Verification items for the finished model (mm, model axes). Face numbers are marked on the shaded views. A direction names the side the tool comes from. Round coordinates to 2 decimals unless told otherwise and drop trailing zeros. Order: outer loops, then holes, each group sorted by start corner. A loop starts at its lowest first (then second) coordinate and runs counter-clockwise, first axis right, second up. Notation, with made-up numbers: (47, 55.25) -> (63, 55.25) arc R8 ccw to (63, 65.25) -> close; hole circle Ø11 at (69.25, 81). An arc over 180 degrees is marked (long way). Return JSON: item names as keys, results as strings. Group by question number.
Item 1: Sectioned sample at B-B on z = 11.5. Give the number of separate pieces and of enclosed holes in the cut face, plus the area to 3 significant figures.
Item 2: Sectioned sample at D-D on y = -11.5. Record the cut outline in (x, z).
Item 3: Draft check along Y on the marked faces 1, 2 and 3. Enter one of: pulls with the +Y half, pulls with the -Y half, needs draft (parallel to the pull), parting line crosses it, or undercut.
Item 4: Access from +Z, -Z, +X, -X, +Y, -Y to the whole of each face (thin tool, end or side, straight path). Record for the marked faces 4 and 5.
Item 5: Sectioned sample at C-C on y = -6. Record the cut outline in (x, z).
Item 6: Sectioned sample at A-A on x = -2. Record the cut outline in (y, z), plus the area to 3 significant figures.
Item 7: Depth check by flat-ended pin: pin 1 Ø2 at (y, z) = (9.5, 6) entering from +X; pin 2 Ø1 at (x, z) = (-8.5, 11) entering from -Y; pin 3 Ø2 at (x, z) = (-11.5, 11.5) entering from -Y. Enter the tip coordinate at first touch or a pass-through.
Item 8: Scan lines: probe 1 along Y at (x, z) = (6.5, 6); probe 2 along Y at (x, z) = (-2, 10); probe 3 along X at (y, z) = (-7.5, 7.75). Record each from-to range of solid material in increasing order. Write a range as from..to.
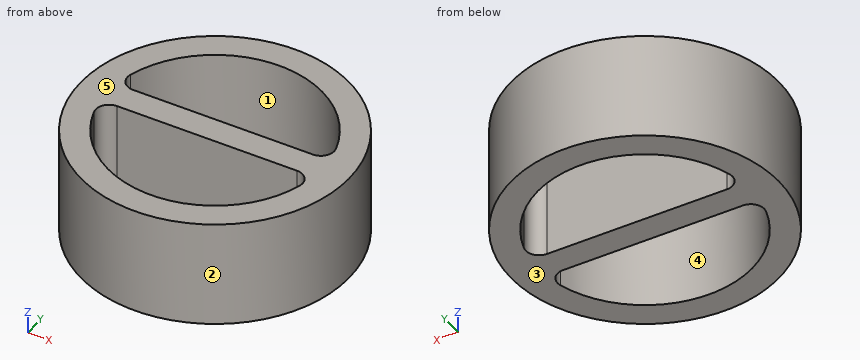
```python
from build123d import *

# Parameters (mm, degrees)
F1_DEPTH = 12.7


with BuildPart() as f1:
    # F0 (on Top) → F1 (new body)
    with BuildSketch(Plane.XY):
        with BuildLine():
            Line((-15.875, 0), (15.875, 0))
            ThreePointArc((15.875, 0), (0, 15.875), (-15.875, 0))
        make_face()
        with BuildLine():
            Line((10.649274, 1.5875), (-10.649274, 1.5875))
            ThreePointArc((-10.649274, 1.5875), (-11.922105, 2.226287), (-12.170599, 3.628571))
            ThreePointArc((-12.170599, 3.628571), (0, 12.7), (12.170599, 3.628571))
            ThreePointArc((12.170599, 3.628571), (11.922105, 2.226287), (10.649274, 1.5875))
        make_face(mode=Mode.SUBTRACT)
        with BuildLine():
            ThreePointArc((-15.875, 0), (0, -15.875), (15.875, 0))
            Line((15.875, 0), (-15.875, 0))
        make_face()
        with BuildLine():
            ThreePointArc((12.170599, -3.628571), (0, -12.7), (-12.170599, -3.628571))
            ThreePointArc((-12.170599, -3.628571), (-11.922105, -2.226287), (-10.649274, -1.5875))
            Line((-10.649274, -1.5875), (10.649274, -1.5875))
            ThreePointArc((10.649274, -1.5875), (11.922105, -2.226287), (12.170599, -3.628571))
        make_face(mode=Mode.SUBTRACT)
    extrude(amount=F1_DEPTH)


solid = f1.part
```
Recorded:
{
 "1": {"separate pieces": "1", "enclosed holes": "2", "area": "369 mm²"},
 "2": {"outline": "(-10.94, 0) -> (-5.39, 0) -> (-5.39, 12.7) -> (-10.94, 12.7) -> close; (5.39, 0) -> (10.94, 0) -> (10.94, 12.7) -> (5.39, 12.7) -> close"},
 "3": {"face 1": "undercut", "face 2": "parting line crosses it", "face 3": "needs draft"},
 "4": {"face 4": "+Z, -Z", "face 5": "+Z, +X, -X, +Y, -Y"},
 "5": {"outline": "(-14.7, 0) -> (-11.19, 0) -> (-11.19, 12.7) -> (-14.7, 12.7) -> close; (11.19, 0) -> (14.7, 0) -> (14.7, 12.7) -> (11.19, 12.7) -> close"},
 "6": {"outline": "(-15.75, 0) -> (-12.54, 0) -> (-12.54, 12.7) -> (-15.75, 12.7) -> close; (-1.59, 0) -> (1.59, 0) -> (1.59, 12.7) -> (-1.59, 12.7) -> close; (12.54, 0) -> (15.75, 0) -> (15.75, 12.7) -> (12.54, 12.7) -> close", "area": "122 mm²"},
 "7": {"pin 1": "x = 13.41", "pin 2": "y = -13.71", "pin 3": "y = -11.91"},
 "8": {"probe 1": "-14.48..-10.91, -1.59..1.59, 10.91..14.48", "probe 2": "-15.75..-12.54, -1.59..1.59, 12.54..15.75", "probe 3": "-13.99..-10.25, 10.25..13.99"}
}
